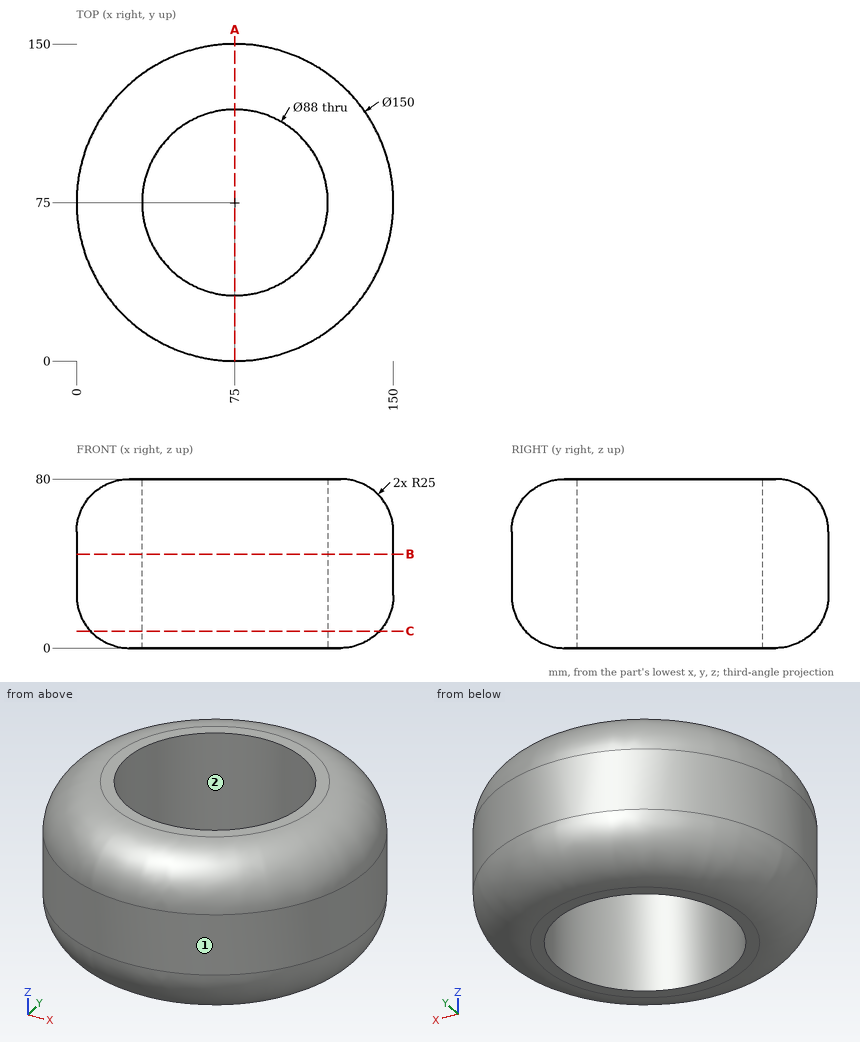
Check sheet for the drawn part. Datum: minimum x, y, z corner. Units: mm. Give positions to 0.01 mm unless a question says otherwise; leave off trailing zeros. Order: outer loops, then holes, each group sorted by start corner. A loop starts at its lowest first (then second) coordinate and runs counter-clockwise, first axis right, second up. Notation, with made-up numbers: (52, 82.25) -> (84, 82.25) arc R14 ccw to (84, 107.25) -> close; hole circle Ø7 at (14, -26.5). An arc over 180 degrees is marked (long way). Use a Markdown table: item, result.
1) Material ranges on probe 1 along Y at (x, z) = (75, 36); probe 2 along Y at (x, z) = (115, 55); probe 3 along X at (y, z) = (89.5, 45), recorded low to high.
Results:
| item | result |
|---|---|
| probe 1 | 0 to 31, 119 to 150 |
| probe 2 | 11.56 to 56.67, 93.33 to 138.44 |
| probe 3 | 1.42 to 33.46, 116.54 to 148.58 |
2) Section check B-B, the plane z = 44.5. Record the boundary of the cut face in (x, y).
Results:
| item | result |
|---|---|
| outline | circle Ø150 at (75, 75); hole circle Ø88 at (75, 75) |
3) Section check A-A, the plane x = 75. Record the boundary of the cut face in (y, z).
Results:
| item | result |
|---|---|
| outline | (0, 25) arc R25 ccw to (25, 0) -> (31, 0) -> (31, 80) -> (25, 80) arc R25 ccw to (0, 55) -> close; (119, 0) -> (125, 0) arc R25 ccw to (150, 25) -> (150, 55) arc R25 ccw to (125, 80) -> (119, 80) -> close |
4) Mould release check, pull along Y, two halves, no side actions. Record for the marked faces 1 and 2: pulls with the +Y half, pulls with the -Y half, needs draft (parallel to the pull), parting line crosses it, or undercut.
Results:
| item | result |
|---|---|
| face 1 | parting line crosses it |
| face 2 | undercut |
5) Section check C-C, the plane z = 8. Record the boundary of the cut face in (x, y).
Results:
| item | result |
|---|---|
| outline | circle Ø136.66 at (75, 75); hole circle Ø88 at (75, 75) |
6) Depth check by flat-ended pin: pin 1 Ø12 at (y, z) = (84.5, 23) entering from -X; pin 2 Ø4 at (y, z) = (48.5, 56.5) entering from +X; pin 3 Ø5 at (y, z) = (116, 32.5) entering from -X. Enter the tip coordinate at first touch or a pass-through.
Results:
| item | result |
|---|---|
| pin 1 | x = 0.1 |
| pin 2 | x = 145.85 |
| pin 3 | x = 10.64 |
